Verification items for the finished model (mm, model axes). A direction names the side the tool comes from. Give positions to 0.01 mm unless a question says otherwise; leave off trailing zeros. Loops run counter-clockwise (first coordinate to the right, second up) from the corner with the lowest first, then second, coordinate; pieces in that order, holes last. Notation, with made-up numbers: (-31.75, 67.25) -> (17.25, 67.25) arc R35 cw to (17.25, 105.25) -> close; hole circle Ø1 at (48.5, 78). An arc over 180 degrees is marked (long way). Use one line per item in the form item = value. Start each with the question number.
from build123d import *

# Parameters (mm, degrees)
F0_W     = 38.1
F0_H     = 38.1
F1_DEPTH = 327.5076
F2_W     = 12.7
F2_H     = 38.1
F3_DEPTH = 50.8
F4_F1_R  = 5.08
F4_F2_R  = 5.08


with BuildPart() as f1:
    # F0 (on Top) → F1 (new body)
    with BuildSketch(Plane.XY):
        with Locations((19.05, -19.05)):
            Rectangle(F0_W, F0_H)
    extrude(amount=F1_DEPTH)

    # F2 (on face) → F3 (cut)
    with BuildSketch(Plane.XY.offset(327.5076)):
        with Locations((19.05, -19.05)):
            Rectangle(F2_W, F2_H)
    extrude(amount=-F3_DEPTH, mode=Mode.SUBTRACT)

    # F4: fillet of radius 5.08 on 4 edges, made by hand

    # F4_f1
    f4_f1_edges = [f1.edges().sort_by_distance(p)[0] for p in [
        (12.7, -19.05, 276.7076),
        (25.4, -19.05, 276.7076),
    ]]
    fillet(f4_f1_edges, radius=F4_F1_R)

    # F4_f2
    f4_f2_edges = [f1.edges().sort_by_distance(p)[0] for p in [
        (19.05, 0, 276.7076),
        (19.05, -38.1, 276.7076),
        (14.1878975516, -38.1, 278.1954975516),
        (23.9121024484, -38.1, 278.1954975516),
        (23.9121024484, 0, 278.1954975516),
        (14.1878975516, 0, 278.1954975516),
    ]]
    fillet(f4_f2_edges, radius=F4_F2_R)


solid = f1.part
Item 1: Tool access check on faces 1 (the cylindrical face through (19.07, -36.65, 275.18)), 2 (the cylindrical face through (23.951, -18.854, 278.235)), 3 (the cylindrical face through (26.849, -1.528, 304.968)). Record the directions out of +Z, -Z, +X, -X, +Y, -Y that give a thin tool (end or side, any length) a straight path to the whole face; none if there is none.
Item 2: Sectioned sample at A-A, the plane z = 303. Enter the section's corners in (x, y).
Item 3: Material ranges on line 1 (Z direction, x = 19.5, y = -15); line 2 (X direction, y = -13.5, z = 289); line 3 (Z direction, x = 16.5, y = -19), recorded low to high.
Item 4: Draft check along X on faces 4 (the flat face through (32, -19, 327.508)), 5 (the flat face through (38.1, -19, 161)), 6 (the cylindrical face through (11.172, -36.651, 304.328)), 7 (the cylindrical face through (26.928, -36.651, 304.968)). Enter one of: +X half, -X half, draft (parallel to the pull), parting line (faces both ways), or undercut.
Item 5: Sectioned sample at B-B, the plane y = -26.5. Enter the section's corners in (x, z), and give its area (3 significant figures).
Item 6: Gauge pin test, flat ends, axial feed: pin 1 Ø4 at (x, y) = (33, -28.5) entering from -Z; pin 2 Ø2 at (x, y) = (19, -12) entering from +Z; pin 3 Ø3 at (x, y) = (23.5, -33) entering from +Z. Record the tip position at first contact, or that the pin passes through.
Outcome:
q1.face_1 = +Z, -Y
q1.face_2 = +Z, +Y, -Y
q1.face_3 = +Z, +Y
q2.outline = (0, -38.1) -> (7.62, -38.1) arc R5.08 ccw to (12.7, -33.02) -> (12.7, -5.08) arc R5.08 ccw to (7.62, 0) -> (0, 0) -> close; (25.4, -33.02) arc R5.08 ccw to (30.48, -38.1) -> (38.1, -38.1) -> (38.1, 0) -> (30.48, 0) arc R5.08 ccw to (25.4, -5.08) -> close
q3.line_1 = 0 to 276.71
q3.line_2 = 0 to 12.7, 25.4 to 38.1
q3.line_3 = 0 to 276.87
q4.face_4 = draft
q4.face_5 = +X half
q4.face_6 = undercut
q4.face_7 = undercut
q5.outline = (0, 0) -> (38.1, 0) -> (38.1, 327.51) -> (25.4, 327.51) -> (25.4, 281.79) arc R5.08 cw to (20.32, 276.71) -> (17.78, 276.71) arc R5.08 cw to (12.7, 281.79) -> (12.7, 327.51) -> (0, 327.51) -> close
q5.area = 11,800 mm^2
q6.pin_1 = 0
q6.pin_2 = 276.71
q6.pin_3 = 279.81
